```python
from build123d import *

# Parameters (mm, degrees)
SKETCH1_R           = 8
BOSS_EXTRUDE1_DEPTH = 58
SKETCH2_OUTSIDE_W   = 30.452
SKETCH2_OUTSIDE_H   = 30.452
SKETCH2_OUTSIDE_R   = 7
CUT_EXTRUDE1_DEPTH  = 1


with BuildPart() as part:
    # Sketch1 → Boss-Extrude1 (new body)
    with BuildSketch(Plane.XY):
        with Locations(Location((0, 0, 0), (0, 0, 180))):
            Circle(SKETCH1_R)
    extrude(amount=BOSS_EXTRUDE1_DEPTH)

    # Sketch2 outside → Cut-Extrude1 (cut)
    with BuildSketch(Plane.XY.offset(56)):
        Rectangle(SKETCH2_OUTSIDE_W, SKETCH2_OUTSIDE_H)
        Circle(SKETCH2_OUTSIDE_R, mode=Mode.SUBTRACT)
    cut_extrude1 = extrude(amount=-CUT_EXTRUDE1_DEPTH, mode=Mode.SUBTRACT)

    # Mirror1: Cut-Extrude1 across plane
    add(cut_extrude1.mirror(Plane.XY.offset(29)), mode=Mode.SUBTRACT)


solid = part.part
```
Check sheet for the modelled part. Datum: model origin and axes. Units: mm. A direction names the side the tool comes from. Give positions to 0.01 mm unless a question says otherwise; leave off trailing zeros. Loops run counter-clockwise (first coordinate to the right, second up) from the corner with the lowest first, then second, coordinate; pieces in that order, holes last. Notation, with made-up numbers: M 15,-15.75 L 47,-15.75 A31 cw 47,15.25 Z; hole C 31,-21.5 d9. An arc over 180 degrees is marked long. Answer as CSV lines item,"result".
Item 1: Sectioned sample at C-C, the plane z = 49. Enter the section's corners in (x, y).
Reply:
outline,"C 0,0 d16"
Item 2: Sectioned sample at B-B, the plane y = 4.25. Enter the section's corners in (x, z), then the cut area to 3 significant figures.
Reply:
outline,"M -6.78,0 L 6.78,0 L 6.78,2 L 5.56,2 L 5.56,3 L 6.78,3 L 6.78,55 L 5.56,55 L 5.56,56 L 6.78,56 L 6.78,58 L -6.78,58 L -6.78,56 L -5.56,56 L -5.56,55 L -6.78,55 L -6.78,3 L -5.56,3 L -5.56,2 L -6.78,2 Z"
area,"781 mm^2"
Item 3: Draft check along Z on faces 3 (the face through (0, 0, 58)), 4 (the face through (0, 0, 0)), 5 (the face through (4, -6, 55)). Enter one of: pulls with the +Z half, pulls with the -Z half, needs draft (parallel to the pull), parting line crosses it, or undercut.
Reply:
face 3,"pulls with the +Z half"
face 4,"pulls with the -Z half"
face 5,"undercut"
Item 4: Sectioned sample at A-A, the plane x = 3.5. Enter the section's corners in (y, z).
Reply:
outline,"M -7.19,0 L 7.19,0 L 7.19,2 L 6.06,2 L 6.06,3 L 7.19,3 L 7.19,55 L 6.06,55 L 6.06,56 L 7.19,56 L 7.19,58 L -7.19,58 L -7.19,56 L -6.06,56 L -6.06,55 L -7.19,55 L -7.19,3 L -6.06,3 L -6.06,2 L -7.19,2 Z"
Item 5: Depth check by flat-ended pin: pin 1 Ø3 at (y, z) = (5.5, 50.5) entering from +X; pin 2 Ø5 at (y, z) = (-5.5, 40) entering from +X; pin 3 Ø3 at (y, z) = (-6, 44) entering from -X; pin 4 Ø1 at (x, y) = (5, 4.5) entering from -Z. Enter the tip coordinate at first touch or a pass-through.
Reply:
pin 1,"x = 6.93"
pin 2,"x = 7.42"
pin 3,"x = -6.61"
pin 4,"z = 0"
Item 6: Set-up check for faces 1 (the face through (1.73, 7.81, 28.64)), 2 (the face through (6.466, -2.681, 55.507)): record each of +Z, -Z, +X, -X, +Y, -Y from which the full face is reachable in a straight line by a thin tool's end or side.
Reply:
face 1,"+Z, -Z"
face 2,"none"
Item 7: Scan lines: L1, parallel to Z at x = 4.75, y = -5.75; L2, parallel to X at y = -3, z = 9.5; L3, parallel to X at y = -3.25, z = 55.5. Record each from-to range of solid material in increasing order.
Reply:
L1,"0 to 2, 3 to 55, 56 to 58"
L2,"-7.42 to 7.42"
L3,"-6.2 to 6.2"
